Autodesk Inventor part; units mm, degrees
ref_plane "YZ Plane" through (0, 0, 0) normal (1, 0, 0) x (0, 1, 0)
ref_plane "XZ Plane" through (0, 0, 0) normal (0, 1, 0) x (-1, 0, 0)
ref_plane "XY Plane" through (0, 0, 0) normal (0, 0, 1) x (1, 0, 0)
sketch "Esquisse1" plane through (0, 0, 0) normal (0, 0, 1) x (1, 0, 0)
  line L0 (-1000, -350) -> (1000, -350)
  line L1 (1000, -350) -> (1000, 350)
  line L2 (1000, 350) -> (-1000, 350)
  line L3 (-1000, 350) -> (-1000, -350)
  line L4 (-1000, -350) -> (1000, 350) construction
  line L5 (1000, -350) -> (-1000, 350) construction
  point P0 (0, 0)
  dimension "d0" = 2000
  dimension "d1" = 700
extrude "Extrusion1" add sketch "Esquisse1" along normal blind 500
sketch "Esquisse3" plane through (0, 0, 0) normal (0, 0, -1) x (-1, 0, 0)
  line L0 (-950, 125) -> (-366.6667, 125)
  line L1 (-366.6667, 125) -> (-366.6667, 300)
  line L2 (-366.6667, 300) -> (-950, 300)
  line L3 (-950, 300) -> (-950, 125)
  line L4 (-1000, 350) -> (1000, 350)
  line L5 (-1000, -350) -> (-1000, 350)
  point P0 (0, 0)
  dimension "d4" = 175
  dimension "d5" = 583.3333
  dimension "d6" = 50
  dimension "d7" = 50
extrude "Extrusion2" cut sketch "Esquisse3" against normal through all
pattern_linear "Réseau rectangulaire1" count 3 spacing 650 along (-1, 0, 0) of "Extrusion2"
pattern_linear "Réseau rectangulaire2" count 3 spacing 215 along (0, -1, 0) of "Extrusion2", "Réseau rectangulaire1"
properties part number "1420-14-06 Meuble noir" material "Bois (bouleau)"
Source: CAD feature listing. Evaluate the final solid. Frame: model axes, mm. A direction names the side the tool comes from. Coordinates: 2 decimals unless noted, no trailing zeros. Loops run counter-clockwise (first coordinate to the right, second up) from the corner with the lowest first, then second, coordinate; pieces in that order, holes last. Notation, with made-up numbers: (48.5, 40.25) - (63.5, 40.25) arc R32 cw to (63.5, 66.25) - close; hole circle Ø2 at (4, 35.5). An arc over 180 degrees is marked (long way). One line per item, written item: value. Start each with the question number.
1. Section C-C (z = 248.5). State how many separate pieces and enclosed holes the cut face has, and give its area (3 significant figures).
2. Section B-B (x = -93.5). Return the cut outline in (y, z), and give its area (3 significant figures).
3. Section A-A (y = 176.5). Return the cut outline in (x, z).
4. Mould query, pull axis X, two halves, no side actions, for faces 1 (the flat face through (-5, 105, 500)), 2 (the flat face through (-646, 85, 246)), 3 (the flat face through (662, -305, 246)). Classes: pulls with the +X half, pulls with the -X half, needs draft (parallel to the pull), parting line crosses it, or undercut.
5. Set-up query: faces 4 (the flat face through (654, 300, 246)), 5 (the flat face through (-14, -350, 246)). Return all of +Z, -Z, +X, -X, +Y, -Y with unobstructed straight access to the full face (end or side cutting, diameter ignored); none if empty.
6. Ray query, L1, parallel to Y at x = -11, z = 178.5; L2, parallel to X at y = -279, z = 414.5. Return the intervals inside material, ascending.
Verdict:
1. separate pieces: 1
1. enclosed holes: 9
1. area: 481,000 mm2
2. outline: (-350, 0) - (-305, 0) - (-305, 500) - (-350, 500) - close; (-130, 0) - (-90, 0) - (-90, 500) - (-130, 500) - close; (85, 0) - (125, 0) - (125, 500) - (85, 500) - close; (300, 0) - (350, 0) - (350, 500) - (300, 500) - close
2. area: 87,500 mm2
3. outline: (-1000, 0) - (-933.33, 0) - (-933.33, 500) - (-1000, 500) - close; (-350, 0) - (-283.33, 0) - (-283.33, 500) - (-350, 500) - close; (300, 0) - (366.67, 0) - (366.67, 500) - (300, 500) - close; (950, 0) - (1000, 0) - (1000, 500) - (950, 500) - close
4. face 1: needs draft
4. face 2: undercut
4. face 3: undercut
5. face 4: +Z, -Z
5. face 5: +Z, -Z, +X, -X, -Y
6. L1: y = -350 to -305, -130 to -90, 85 to 125, 300 to 350
6. L2: x = -1000 to -933.33, -350 to -283.33, 300 to 366.67, 950 to 1000
